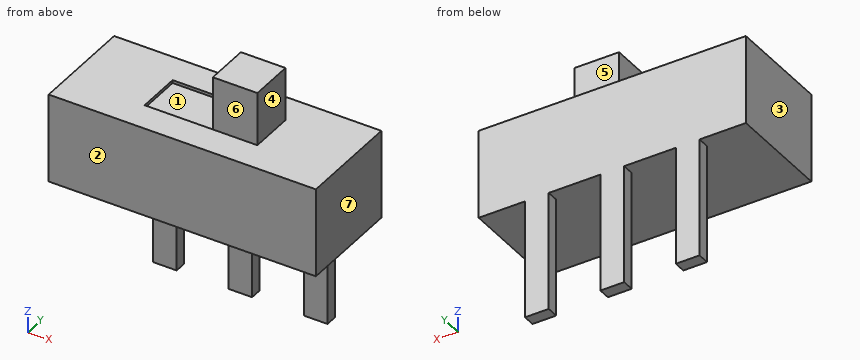
```python
from build123d import *

# Parameters (mm, degrees)
SKETCH_1_W          = 9
SKETCH_1_H          = 3
EXTRUDE_1_DEPTH     = 3.5
SKETCH_2_W          = 3.8
SKETCH_2_H          = 1.5
CUT_EXTRUDE_1_DEPTH = 0.1
SKETCH_3_W          = 1.5
SKETCH_3_H          = 1.5
EXTRUDE_2_DEPTH     = 1.9
SKETCH_4_W          = 0.8
SKETCH_4_H          = 0.4
EXTRUDE_3_DEPTH     = 4


with BuildPart() as part:
    # Эскиз1 → Бобышка-Вытянуть1 (new body)
    with BuildSketch(Plane(origin=(0, 0, 0), x_dir=(1, 0, 0), z_dir=(0, 1, 0))):
        Rectangle(SKETCH_1_W, SKETCH_1_H)
    extrude(amount=EXTRUDE_1_DEPTH)

    # Эскиз2 → Вырез-Вытянуть1 (cut)
    with BuildSketch(Plane.XY.offset(1.5)):
        with Locations((0, 1.75)):
            Rectangle(SKETCH_2_W, SKETCH_2_H)
    extrude(amount=-CUT_EXTRUDE_1_DEPTH, mode=Mode.SUBTRACT)

    # Эскиз3 → Бобышка-Вытянуть2 (add)
    with BuildSketch(Plane.XY.offset(1.4)):
        with Locations((1.15, 1.75)):
            Rectangle(SKETCH_3_W, SKETCH_3_H)
    extrude(amount=EXTRUDE_2_DEPTH)

    # Эскиз4 → Бобышка-Вытянуть3 (add)
    with BuildSketch(Plane(origin=(0, 0, -1.5), x_dir=(-1, 0, 0), z_dir=(0, 0, -1))):
        with Locations((-2.54, 3.3)):
            Rectangle(SKETCH_4_W, SKETCH_4_H)
        with Locations((0, 3.3)):
            Rectangle(SKETCH_4_W, SKETCH_4_H)
        with Locations((2.54, 3.3)):
            Rectangle(SKETCH_4_W, SKETCH_4_H)
    extrude(amount=EXTRUDE_3_DEPTH)


solid = part.part
```
Work out the finished part from the listing and answer in its coordinate system (mm). Face numbers are marked on the shaded views. A direction names the side the tool comes from. Round coordinates to 2 decimals unless told otherwise and drop trailing zeros. Loops run counter-clockwise (first coordinate to the right, second up) from the corner with the lowest first, then second, coordinate; pieces in that order, holes last.
(1) The part is cut by section B-B, the plane x = -1.75. Give the vertices of the cut face in (y, z), and give its area (4 significant figures).
Computed values:
outline: (0, -1.5) - (3.5, -1.5) - (3.5, 1.5) - (2.5, 1.5) - (2.5, 1.4) - (1, 1.4) - (1, 1.5) - (0, 1.5) - close
area: 10.35 mm2
(2) The part is cut by section C-C, the plane y = 3.3. Give the vertices of the cut face in (x, z).
Computed values:
outline: (-4.5, -1.5) - (-2.94, -1.5) - (-2.94, -5.5) - (-2.14, -5.5) - (-2.14, -1.5) - (-0.4, -1.5) - (-0.4, -5.5) - (0.4, -5.5) - (0.4, -1.5) - (2.14, -1.5) - (2.14, -5.5) - (2.94, -5.5) - (2.94, -1.5) - (4.5, -1.5) - (4.5, 1.5) - (-4.5, 1.5) - close
(3) The part is cut by section A-A, the plane z = -3. Give the vertices of the cut face in (x, y).
Computed values:
outline: (-2.94, 3.1) - (-2.14, 3.1) - (-2.14, 3.5) - (-2.94, 3.5) - close; (-0.4, 3.1) - (0.4, 3.1) - (0.4, 3.5) - (-0.4, 3.5) - close; (2.14, 3.1) - (2.94, 3.1) - (2.94, 3.5) - (2.14, 3.5) - close
(4) For the marked faces 5, 6 and 7, determine the directions among +Z, -Z, +X, -X, +Y, -Y from which every point of the face is accessible in a straight line to the end or side of a thin tool.
Computed values:
face 5: +Z, +X, -X, +Y
face 6: +Z, +X, -X, -Y
face 7: +Z, -Z, +X, +Y, -Y
(5) The mould has two halves that part along X. Classify the marked faces 1, 2, 3 and 4: pulls with the +X half, pulls with the -X half, needs draft (parallel to the pull), parting line crosses it, or undercut.
Computed values:
face 1: undercut
face 2: needs draft
face 3: pulls with the -X half
face 4: pulls with the +X half
(6) The part is cut by section D-D, the plane z = 2.75. Give the vertices of the cut face in (x, y).
Computed values:
outline: (0.4, 1) - (1.9, 1) - (1.9, 2.5) - (0.4, 2.5) - close
(7) Each of these flat-tipped pins is pushed along its axis until it touches: P1, Ø1.2, axis at x = -0.5, y = 2, coming from the +Z side; P2, Ø0.8, axis at y = 1.5, z = 2.5, coming from the +X side; P3, Ø0.8, axis at x = 1, z = 2, coming from the +Y side. Where does it stop, or does it pass through?
Computed values:
P1: stops at z = 1.5
P2: stops at x = 1.9
P3: stops at y = 2.5
(8) Find the intervals of material crossed by L1, parallel to Z at x = 1.5, y = 3; L2, parallel to Y at x = -2.75, z = -3.75; L3, parallel to Z at x = 1, y = 1.35, in increasing order.
Computed values:
L1: z = -1.5 to 1.5
L2: y = 3.1 to 3.5
L3: z = -1.5 to 3.3
